```python
from build123d import *

# Parameters (mm, degrees)
F0_R     = 38.1
F0_R_2   = 33.02
F1_DEPTH = 25.4
F2_R     = 38.1
F3_DEPTH = 5.08
F4_R     = 2.599995
F5_DEPTH = 228.6


with BuildPart() as f1:
    # F0 (on Top) → F1 (new body)
    with BuildSketch(Plane.XY):
        Circle(F0_R)
        Circle(F0_R_2, mode=Mode.SUBTRACT)
    extrude(amount=F1_DEPTH)

    # F2 (on face) → F3 (join)
    with BuildSketch(Plane.XY.offset(25.4)):
        Circle(F2_R)
    extrude(amount=F3_DEPTH)

    # F4 (on face) → F5 (cut)
    with BuildSketch(Plane(origin=(0, 0, 25.4), x_dir=(1, 0, 0), z_dir=(0, 0, -1))):
        Circle(F4_R)
    extrude(amount=-F5_DEPTH, mode=Mode.SUBTRACT)


solid = f1.part
```
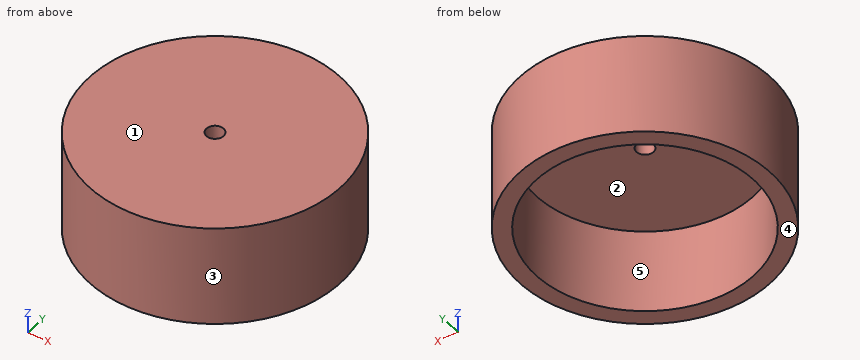
For this review, take the finished solid that the model builds, in its own axes (mm). Face numbers are marked on the shaded views. A direction names the side the tool comes from. Round coordinates to 2 decimals unless told otherwise and drop trailing zeros. Write each loop counter-clockwise with the first axis right and the second up, starting at its lowest first coordinate (ties: lowest second). Pieces come first, ordered by that corner, then holes. Notation, with made-up numbers: M 44.25,-4 L 51.25,-4 A20 cw 51.25,2 Z; hole C -34,-14.5 d3. An arc over 180 degrees is marked long. One line per item, written item: value. Start each with the question number.
(1) Machinability: for the marked faces 1 and 2, which of the approach directions +Z, -Z, +X, -X, +Y, -Y give a long, thin tool a straight path to every point of the face, cutting with its end or side? Answer none if there is none.
(2) The part is to be moulded in two halves that separate along Y. For the marked faces 3, 4 and 5, say which applies: released by +Y, released by -Y, zero draft, split by the parting line, or undercut.
(3) Insertion check: pin 1 (5 mm diameter, centred on y = 5.5, z = 9, fed in from +X); pin 2 (2 mm diameter, centred on y = -12, z = 20, fed in from +X); pin 3 (5 mm diameter, centred on y = -3.5, z = 13.5, fed in from -X). Each pin has a flat end and moves straight along its axis. Give the tip position at first contact, or say it passes through.
(4) We need section A-A (x = 0). Give the boundary of the cut face in (y, z), and give its area (3 significant figures).
(5) We need section C-C (z = 5). Give the boundary of the cut face in (x, y), and give its area (3 significant figures).
(6) Wall thickness on line 1 (Y direction, x = 0, z = 28.1); line 2 (Z direction, x = 6, y = -17); line 3 (X direction, y = 0.5, z = 11): over which ranges is each line inside the solid? List them lowest first.
(7) We need section D-D (y = 21.5). Give the boundary of the cut face in (x, z).
Result:
1. face 1: +Z, +X, -X, +Y, -Y
1. face 2: -Z
2. face 3: split by the parting line
2. face 4: zero draft
2. face 5: undercut
3. pin 1: x = 37.98
3. pin 2: x = 36.48
3. pin 3: x = -38.09
4. outline: M -38.1,0 L -33.02,0 L -33.02,25.4 L -2.6,25.4 L -2.6,30.48 L -38.1,30.48 Z; M 2.6,25.4 L 33.02,25.4 L 33.02,0 L 38.1,0 L 38.1,30.48 L 2.6,30.48 Z
4. area: 619 mm²
5. outline: C 0,0 d76.2; hole C 0,0 d66.04
5. area: 1,140 mm²
6. line 1: -38.1 to -2.6, 2.6 to 38.1
6. line 2: 25.4 to 30.48
6. line 3: -38.1 to -33.02, 33.02 to 38.1
7. outline: M -31.45,0 L -25.06,0 L -25.06,25.4 L 25.06,25.4 L 25.06,0 L 31.45,0 L 31.45,30.48 L -31.45,30.48 Z
